from build123d import *

# Parameters (mm, degrees)
F0_W     = 6
F0_H     = 0.3
F1_DEPTH = 7
F2_R     = 2


with BuildPart() as f1:
    # F0 (on Top) → F1 (new body)
    with BuildSketch(Plane.XY):
        with BuildLine():
            ThreePointArc((-3.6, 7), (-4.185786, 5.585786), (-5.6, 5))
            Line((-5.6, 5), (-3.6, 5))
            Line((-3.6, 5), (-3.6, 7))
        make_face()
        with BuildLine():
            Line((3.6, 7), (3.6, 5))
            Line((3.6, 5), (5.6, 5))
            ThreePointArc((5.6, 5), (4.185786, 5.585786), (3.6, 7))
        make_face()
        with Locations((-20.5, -0.15)):
            Rectangle(F0_W, F0_H)
        Polygon((-5.6, 5), (-23.5, 5), (-23.5, 0), (-17.5, 0), (17.5, 0), (23.5, 0), (23.5, 5), (5.6, 5), (3.6, 5), (3.6, 2.7), (-3.6, 2.7), (-3.6, 5), align=None)
        with Locations((20.5, -0.15)):
            Rectangle(F0_W, F0_H)
    extrude(amount=F1_DEPTH)

    # F2
    f2_edges = [f1.edges().sort_by_distance(p)[0] for p in [
        (-23.5, 5, 3.5),
        (23.5, 5, 3.5),
        (-23.5, -0.3, 3.5),
        (23.5, -0.3, 3.5),
    ]]
    fillet(f2_edges, radius=F2_R)


solid = f1.part
Verification items for the finished model (mm, model axes). A direction names the side the tool comes from. Round coordinates to 2 decimals unless told otherwise and drop trailing zeros. Order: outer loops, then holes, each group sorted by start corner. A loop starts at its lowest first (then second) coordinate and runs counter-clockwise, first axis right, second up.
1. Section check A-A on y = 5.75. Record the cut outline in (x, z).
Final values:
outline: (-4.04, 0) - (-3.6, 0) - (-3.6, 7) - (-4.04, 7) - close; (3.6, 0) - (4.04, 0) - (4.04, 7) - (3.6, 7) - close
2. Section check D-D on y = 4. Record the cut outline in (x, z).
Final values:
outline: (-23.23, 0) - (-3.6, 0) - (-3.6, 7) - (-23.23, 7) - close; (3.6, 0) - (23.23, 0) - (23.23, 7) - (3.6, 7) - close
3. Section check B-B on z = 2.75. Record the cut outline in (x, y), then the cut area to 3 significant figures.
Final values:
outline: (-23.5, 1.7) arc R2 ccw to (-21.5, -0.3) - (-17.5, -0.3) - (-17.5, 0) - (17.5, 0) - (17.5, -0.3) - (21.5, -0.3) arc R2 ccw to (23.5, 1.7) - (23.5, 3) arc R2 ccw to (21.5, 5) - (5.6, 5) arc R2 cw to (3.6, 7) - (3.6, 2.7) - (-3.6, 2.7) - (-3.6, 7) arc R2 cw to (-5.6, 5) - (-21.5, 5) arc R2 ccw to (-23.5, 3) - close
area: 220 mm2
4. Section check C-C on x = -13.5. Record the cut outline in (y, z).
Final values:
outline: (0, 0) - (5, 0) - (5, 7) - (0, 7) - close
5. Release check for a two-part mould opening along X. For faces 4 (the flat face through (3.6, 5, 3)), 5 (the cylindrical face through (-22.93, 0.3, 3.55)), 6 (the cylindrical face through (22.93, 4.4, 3.55)) record: +X half, -X half, draft (parallel to the pull), parting line (faces both ways), or undercut.
Final values:
face 4: undercut
face 5: -X half
face 6: +X half
6. Thickness scan on L1, parallel to Y at x = 15, z = 1; L2, parallel to Y at x = -20.5, z = 4; L3, parallel to X at y = 4.75, z = 5.5. Record the ranges inside material, lowest first.
Final values:
L1: y = 0 to 5
L2: y = -0.3 to 5
L3: x = -22.47 to -3.6, 3.6 to 22.47
7. Go/stop test with flat-tipped pins: P1, Ø3.5, axis at x = -1.5, z = 3, coming from the +Y side; P2, Ø1.3, axis at y = 4, z = 4, coming from the -X side; P3, Ø3.5, axis at y = 6, z = 5, coming from the +X side. Record where each tip stops, or that it passes through.
Final values:
P1: stops at y = 2.7
P2: stops at x = -23.47
P3: stops at x = 23.06
8. Access from +Z, -Z, +X, -X, +Y, -Y to the whole of each face (thin tool, end or side, straight path). Record for faces 1 (the flat face through (0, 0, 3)), 2 (the flat face through (-13, 5, 3)), 3 (the flat face through (14, 5, 3)).
Final values:
face 1: +Z, -Z, -Y
face 2: +Z, -Z, -X, +Y
face 3: +Z, -Z, +X, +Y
